Study the drawing (mm; zero at the part's minimum x, y, z) and answer. Coordinates: 2 decimals unless noted, no trailing zeros. Write each loop counter-clockwise with the first axis right and the second up, starting at its lowest first coordinate (ties: lowest second). Pieces come first, ordered by that corner, then holes. Notation, with made-up numbers: (-3.5, 84.25) -> (9.5, 84.25) arc R23 ccw to (9.5, 112.25) -> close; hole circle Ø10 at (70.25, 14.5). An arc over 180 degrees is marked (long way). Answer in a Markdown table with one row per item. Add a question column.
Item 1: Straight lines are drawn through the part: line 1 (Y direction, x = 17, z = 0.4); line 2 (Y direction, x = 15, z = 0.3); line 3 (Y direction, x = 13, z = 0.85) (1 decimal). For each, find the intervals that lie inside material, in ascending order. Write a range as from..to.
Item 2: Section D-D on x = 11 is taken. Write down the section's boundary in (y, z).
Item 3: Section A-A on y = 44.5 is taken. Write down the section's boundary in (x, z) (1 decimal).
Item 4: Section B-B on x = 16 is taken. Write down the section's boundary in (y, z).
Item 5: Section C-C on z = 0.4 is taken. Count the separate pieces of the cut face and the enclosed holes in it, then the cut area to 3 significant figures.
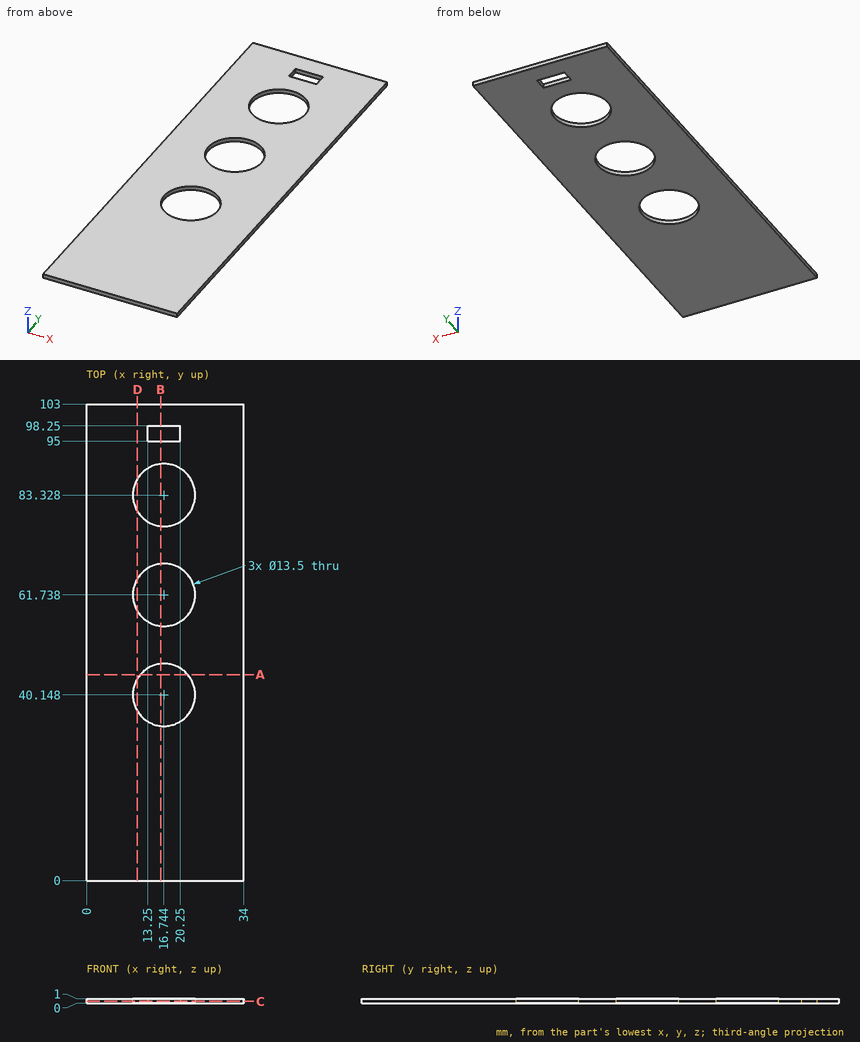
Results below:
| question | item | result |
|---|---|---|
| 1 | line 1 | y = 0..33.4, 46.89..54.99, 68.48..76.58, 90.07..95, 98.25..103 |
| 1 | line 2 | y = 0..33.63, 46.67..55.22, 68.26..76.81, 89.85..95, 98.25..103 |
| 1 | line 3 | y = 0..34.5, 45.8..56.1, 67.4..77.7, 88.9..103 |
| 2 | outline | (0, 0) -> (36.6, 0) -> (36.6, 1) -> (0, 1) -> close; (43.69, 0) -> (58.19, 0) -> (58.19, 1) -> (43.69, 1) -> close; (65.28, 0) -> (79.78, 0) -> (79.78, 1) -> (65.28, 1) -> close; (86.87, 0) -> (103, 0) -> (103, 1) -> (86.87, 1) -> close |
| 3 | outline | (0, 0) -> (11.6, 0) -> (11.6, 1) -> (0, 1) -> close; (21.9, 0) -> (34, 0) -> (34, 1) -> (21.9, 1) -> close |
| 4 | outline | (0, 0) -> (33.44, 0) -> (33.44, 1) -> (0, 1) -> close; (46.86, 0) -> (55.03, 0) -> (55.03, 1) -> (46.86, 1) -> close; (68.45, 0) -> (76.62, 0) -> (76.62, 1) -> (68.45, 1) -> close; (90.04, 0) -> (95, 0) -> (95, 1) -> (90.04, 1) -> close; (98.25, 0) -> (103, 0) -> (103, 1) -> (98.25, 1) -> close |
| 5 | separate pieces | 1 |
| 5 | enclosed holes | 4 |
| 5 | area | 3,050 mm2 |
